```python
from build123d import *

# Parameters (mm, degrees)
SKETCH1_W             = 177.8
SKETCH1_H             = 88.9
SKETCH1_R             = 6.35
BOSS_EXTRUDE1_DEPTH   = 5.08
F_6_CLEARANCE_HOLE1_D = 3.7973


with BuildPart() as part:
    # Sketch1 → Boss-Extrude1 (new body)
    with BuildSketch(Plane.XY):
        Rectangle(SKETCH1_W, SKETCH1_H)
        Circle(SKETCH1_R, mode=Mode.SUBTRACT)
    extrude(amount=BOSS_EXTRUDE1_DEPTH)

    # #6 Clearance Hole1 (through all)
    with Locations(Plane.XY.offset(5.08)):
        with Locations((76.2, -31.75), (-76.2, 31.75), (-76.2, -31.75), (76.2, 31.75), (12.7, -31.75), (-12.7, 31.75), (-12.7, -31.75), (12.7, 31.75)):
            Hole(F_6_CLEARANCE_HOLE1_D / 2)


solid = part.part
```
For this review, take the finished solid that the model builds, in its own axes (mm). Round coordinates to 2 decimals unless told otherwise and drop trailing zeros. Loops run counter-clockwise (first coordinate to the right, second up) from the corner with the lowest first, then second, coordinate; pieces in that order, holes last.
Q1. To check wall thickness, follow line 1 along Y through (x, z) = (76.2, 2.2); line 2 along Y through (x, z) = (0, 2.7); line 3 along Y through (x, z) = (74.5, 1.85). State the ranges of each line that lie inside material, in increasing order.
Result sheet:
line 1: y = -44.45 to -33.65, -29.85 to 29.85, 33.65 to 44.45
line 2: y = -44.45 to -6.35, 6.35 to 44.45
line 3: y = -44.45 to -32.6, -30.9 to 30.9, 32.6 to 44.45
Q2. Add section B-B on y = 31.75. Write out the cut boundary in (x, z).
Result sheet:
outline: (-88.9, 0) - (-78.1, 0) - (-78.1, 5.08) - (-88.9, 5.08) - close; (-74.3, 0) - (-14.6, 0) - (-14.6, 5.08) - (-74.3, 5.08) - close; (-10.8, 0) - (10.8, 0) - (10.8, 5.08) - (-10.8, 5.08) - close; (14.6, 0) - (74.3, 0) - (74.3, 5.08) - (14.6, 5.08) - close; (78.1, 0) - (88.9, 0) - (88.9, 5.08) - (78.1, 5.08) - close
Q3. Add section C-C on y = 0. Write out the cut boundary in (x, z).
Result sheet:
outline: (-88.9, 0) - (-6.35, 0) - (-6.35, 5.08) - (-88.9, 5.08) - close; (6.35, 0) - (88.9, 0) - (88.9, 5.08) - (6.35, 5.08) - close
Q4. Add section A-A on x = 0. Write out the cut boundary in (y, z), plus the area to 3 significant figures.
Result sheet:
outline: (-44.45, 0) - (-6.35, 0) - (-6.35, 5.08) - (-44.45, 5.08) - close; (6.35, 0) - (44.45, 0) - (44.45, 5.08) - (6.35, 5.08) - close
area: 387 mm2
Q5. Mouldability with a two-part tool opening along Y and no side actions: class faces 1 (the face through (-1, 44.45, 3)), 2 (the face through (-1, -44.45, 3)), 3 (the face through (-78.01, -31.18, 2.5)), 4 (the face through (88.9, -1, 3)) as +Y half, -Y half, draft (parallel to the pull), parting line (faces both ways), or undercut.
Result sheet:
face 1: +Y half
face 2: -Y half
face 3: undercut
face 4: draft
Q6. Insertion check: pin 1 Ø2.5 at (x, y) = (76.2, 31.75) entering from -Z. The pin has a flat end and moves straight along its axis. Give the tip position at first contact, or say it passes through.
Result sheet:
pin 1: passes through
